from build123d import *

# Parameters (mm, degrees)
SKETCH10_W          = 2.54
SKETCH10_H          = 5.08
SKETCH10_W_2        = 5.08
SKETCH10_H_2        = 2.54
BOSS_EXTRUDE3_DEPTH = 15.875
BOSS_EXTRUDE4_DEPTH = 31.75
SKETCH12_W          = 13.97
SKETCH12_H          = 7.62
CUT_EXTRUDE1_DEPTH  = 42.639734629
SKETCH14_W          = 31.75
SKETCH14_H          = 38.1
SKETCH14_W_2        = 25.6
SKETCH14_H_2        = 25.6
BOSS_EXTRUDE5_DEPTH = 25.4
CUT_EXTRUDE2_DEPTH  = 25.4


with BuildPart() as part:
    # Sketch10 → Boss-Extrude3 (new, symmetric)
    with BuildSketch(Plane(origin=(0, 0, 0), x_dir=(0, 0, -1), z_dir=(1, 0, 0))):
        with Locations((-11.43, 0)):
            Rectangle(SKETCH10_W, SKETCH10_H)
        with BuildLine():
            Line((-5.08, 2.54), (-9.740509205, 6.542688341))
            ThreePointArc((-9.740509205, 6.542688341), (-10.012022021, 6.580814495), (-10.16, 6.35))
            Line((-10.16, 6.35), (-10.16, -6.35))
            ThreePointArc((-10.16, -6.35), (-10.012022021, -6.580814495), (-9.740509205, -6.542688341))
            Line((-9.740509205, -6.542688341), (-5.08, -2.54))
            Line((-5.08, -2.54), (-5.08, 2.54))
        make_face()
        with BuildLine():
            Line((6.35, 10.16), (-6.35, 10.16))
            ThreePointArc((-6.35, 10.16), (-6.580814495, 10.012022021), (-6.542688341, 9.740509205))
            Line((-6.542688341, 9.740509205), (-2.54, 5.08))
            Line((-2.54, 5.08), (2.54, 5.08))
            Line((2.54, 5.08), (6.542688341, 9.740509205))
            ThreePointArc((6.542688341, 9.740509205), (6.580814495, 10.012022021), (6.35, 10.16))
        make_face()
        with Locations((0, 11.43)):
            Rectangle(SKETCH10_W_2, SKETCH10_H_2)
        with BuildLine():
            ThreePointArc((6.542688341, -9.740509205), (6.580814495, -10.012022021), (6.35, -10.16))
            Line((6.35, -10.16), (-6.35, -10.16))
            ThreePointArc((-6.35, -10.16), (-6.580814495, -10.012022021), (-6.542688341, -9.740509205))
            Line((-6.542688341, -9.740509205), (-2.54, -5.08))
            Line((-2.54, -5.08), (2.54, -5.08))
            Line((2.54, -5.08), (6.542688341, -9.740509205))
        make_face()
        with Locations((0, -11.43)):
            Rectangle(SKETCH10_W_2, SKETCH10_H_2)
        with BuildLine():
            Line((5.08, 2.54), (5.08, -2.54))
            Line((5.08, -2.54), (9.740509205, -6.542688341))
            ThreePointArc((9.740509205, -6.542688341), (10.012022021, -6.580814495), (10.16, -6.35))
            Line((10.16, -6.35), (10.16, -2.54))
            Line((10.16, -2.54), (10.16, 2.54))
            Line((10.16, 2.54), (10.16, 6.35))
            ThreePointArc((10.16, 6.35), (10.012022021, 6.580814495), (9.740509205, 6.542688341))
            Line((9.740509205, 6.542688341), (5.08, 2.54))
        make_face()
        with Locations((11.43, 0)):
            Rectangle(SKETCH10_W, SKETCH10_H)
    extrude(amount=BOSS_EXTRUDE3_DEPTH, both=True)

    # Sketch11 → Boss-Extrude4 (add)
    with BuildSketch(Plane(origin=(15.875, 0, 0), x_dir=(0, 0, -1), z_dir=(1, 0, 0))):
        Polygon((-12.7, -2.54), (-12.7, -12.7), (12.7, -12.7), (12.7, -2.54), (12.7, 2.54), (12.7, 10.16), (19.05, 10.16), (19.05, -19.05), (-19.05, -19.05), (-19.05, 10.16), (-12.7, 10.16), (-12.7, 2.54), align=None)
    extrude(amount=-BOSS_EXTRUDE4_DEPTH)

    # Sketch12 → Cut-Extrude1 (cut, through all)
    with BuildSketch(Plane(origin=(15.875, 0, 0), x_dir=(0, 0, -1), z_dir=(1, 0, 0))):
        with Locations((0, 8.89)):
            Rectangle(SKETCH12_W, SKETCH12_H)
    extrude(amount=-CUT_EXTRUDE1_DEPTH, mode=Mode.SUBTRACT)

    # Sketch14 → Boss-Extrude5 (add)
    with BuildSketch(Plane.XZ.offset(19.05)):
        Rectangle(SKETCH14_W, SKETCH14_H)
        Rectangle(SKETCH14_W_2, SKETCH14_H_2, mode=Mode.SUBTRACT)
    extrude(amount=BOSS_EXTRUDE5_DEPTH)

    # Sketch15 → Cut-Extrude2 (cut)
    with BuildSketch(Plane.XZ.offset(44.45)):
        Polygon((-15.875, -2.5), (-15.875, 2.5), (-2.5, 2.5), (-2.5, 19.05), (2.5, 19.05), (2.5, 2.5), (15.875, 2.5), (15.875, -2.5), (2.5, -2.5), (2.5, -19.05), (-2.5, -19.05), (-2.5, -2.5), align=None)
    extrude(amount=-CUT_EXTRUDE2_DEPTH, mode=Mode.SUBTRACT)


solid = part.part
Can you work these out from the model? Positions are in its coordinate system, mm. A direction names the side the tool comes from. Coordinates: 2 decimals unless noted, no trailing zeros. Order: outer loops, then holes, each group sorted by start corner. A loop starts at its lowest first (then second) coordinate and runs counter-clockwise, first axis right, second up. Notation, with made-up numbers: M 86,70 L 108,70 A12 cw 108,91 Z; hole C 54,89.5 d6. An arc over 180 degrees is marked long. Answer as CSV lines item,"result".
(1) Suppose I cut it at D-D on z = 14. Please give me the cut outline in (x, y) (3 decimals), plus the area to 3 significant figures.
Geometry check:
outline,"M -15.875,-44.45 L -2.5,-44.45 L -2.5,-19.05 L 2.5,-19.05 L 2.5,-44.45 L 15.875,-44.45 L 15.875,10.16 L -15.875,10.16 Z"
area,"1,610 mm^2"
(2) I'm going to push flat-ended pins straight in: pin 1 (2 mm diameter, centred on x = -2, z = 3.5, fed in from +Y); pin 2 (0.8 mm diameter, centred on x = 8, z = -11.5, fed in from -Y); pin 3 (2 mm diameter, centred on x = -5, z = -11, fed in from +Y); pin 4 (12 mm diameter, centred on x = 11.5, z = 0, fed in from -Y). Where does each tip first touch, or does it pass through?
Geometry check:
pin 1,"y = -5.08"
pin 2,"y = -19.05"
pin 3,"y = 6.59"
pin 4,"y = -44.45"
(3) Suppose I cut it at C-C on y = -39.5. Please give me the cut outline in (x, z) (3 decimals), plus the area to 3 significant figures.
Geometry check:
outline,"M -15.875,-19.05 L -2.5,-19.05 L -2.5,-12.8 L -12.8,-12.8 L -12.8,-2.5 L -15.875,-2.5 Z; M -15.875,2.5 L -12.8,2.5 L -12.8,12.8 L -2.5,12.8 L -2.5,19.05 L -15.875,19.05 Z; M 2.5,-19.05 L 15.875,-19.05 L 15.875,-2.5 L 12.8,-2.5 L 12.8,-12.8 L 2.5,-12.8 Z; M 2.5,12.8 L 12.8,12.8 L 12.8,2.5 L 15.875,2.5 L 15.875,19.05 L 2.5,19.05 Z"
area,"461 mm^2"
(4) Suppose I cut it at A-A on y = 0. Please give me the cut outline in (x, z) (3 decimals).
Geometry check:
outline,"M -15.875,-19.05 L 15.875,-19.05 L 15.875,-5.08 L -15.875,-5.08 Z; M -15.875,5.08 L 15.875,5.08 L 15.875,19.05 L -15.875,19.05 Z"
(5) Please list where these lines run through material, in increasing order: L1, parallel to Z at x = -7.5, y = -12.5; L2, parallel to X at y = -26, z = -9 (3 decimals); L3, parallel to Z at x = -11.5, y = -32.5.
Geometry check:
L1,"-19.05 to -12.7, -2.54 to 2.54, 12.7 to 19.05"
L2,"-15.875 to -12.8, 12.8 to 15.875"
L3,"-19.05 to -12.8, 12.8 to 19.05"
(6) On a 3-axis mill with a long thin cutter (end or side, diameter ignored), from which of +Z, -Z, +X, -X, +Y, -Y can I reach the whole of each face in a straight line? I mean faces 4 (the flat face through (0, -11, -2.54)), 5 (the flat face through (-8, -32, 12.8)), 6 (the flat face through (0, 2.54, 11)), 7 (the flat face through (2.5, -32, -16)), 8 (the flat face through (-14, -32, -2.5)). Say none if no direction works.
Geometry check:
face 4,"+X, -X"
face 5,"-Y"
face 6,"+X, -X, +Y"
face 7,"+Z, -Z, -Y"
face 8,"+X, -X, -Y"
(7) Suppose I cut it at B-B on z = -8.5. Please give me the cut outline in (x, y) (3 decimals).
Geometry check:
outline,"M -15.875,-44.45 L -12.8,-44.45 L -12.8,-19.05 L 12.8,-19.05 L 12.8,-44.45 L 15.875,-44.45 L 15.875,-12.7 L -15.875,-12.7 Z; M -15.875,-5.477 L 15.875,-5.477 L 15.875,5.477 L -15.875,5.477 Z"
(8) If we mould it in two halves opening along X, with no side actions, what happens to faces 1 (the flat face through (0, -2.54, -11)), 2 (the flat face through (2.5, -32, 16)), 3 (the flat face through (-15.875, -17, 0))? For each: released by +X, released by -X, zero draft, split by the parting line, or undercut.
Geometry check:
face 1,"zero draft"
face 2,"undercut"
face 3,"released by -X"
